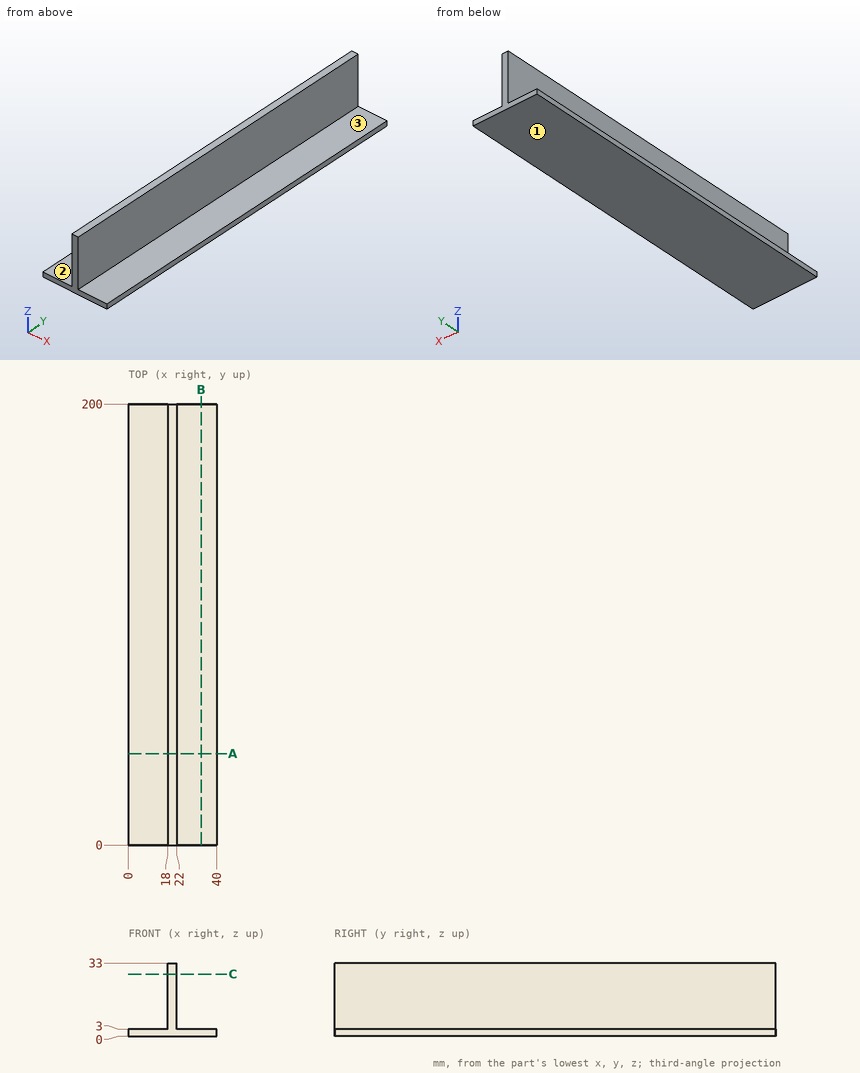
Answer from the drawing. Dimensions are ordinates in mm from the lowest x, y and z of the part. A direction names the side the tool comes from. Coordinates: 2 decimals unless noted, no trailing zeros. Write each loop counter-clockwise with the first axis right and the second up, starting at its lowest first coordinate (ties: lowest second). Pieces come first, ordered by that corner, then holes. Notation, with made-up numbers: M 47.25,41 L 104.25,41 A21 cw 104.25,66 Z; hole C 25,-25 d10. An arc over 180 degrees is marked long. Put each result on its own line as item: value. Start each with the question number.
1. A cutting plane is placed at C-C on z = 28. Write down the section's boundary in (x, y).
2. Consider line 1 (Z direction, x = 36.5, y = 144.5); line 2 (X direction, y = 53, z = 21). Determine where each line is inside the solid, lowest interval first. Write a range as from..to.
3. Which of the six approach directions +Z, -Z, +X, -X, +Y, -Y give full straight-line access (tool end or side, diameter ignored) to the marked faces 1, 2 and 3?
4. A cutting plane is placed at A-A on y = 41.5. Write down the section's boundary in (x, z), then the cut area to 3 significant figures.
5. Flat-ended cylindrical pins translate along their axes: P1, Ø5.5, axis at x = 34.5, y = 125, coming from the +Z side; P2, Ø10, axis at y = 21, z = 23, coming from the -X side. Find the tip coordinate at first contact, or state that the pin passes through.
6. A cutting plane is placed at B-B on x = 33. Write down the section's boundary in (y, z).
Resolved:
1. outline: M 18,0 L 22,0 L 22,200 L 18,200 Z
2. line 1: z = 0..3
2. line 2: x = 18..22
3. face 1: -Z, +X, -X, +Y, -Y
3. face 2: +Z, -X, +Y, -Y
3. face 3: +Z, +X, +Y, -Y
4. outline: M 0,0 L 40,0 L 40,3 L 22,3 L 22,33 L 18,33 L 18,3 L 0,3 Z
4. area: 240 mm2
5. P1: stops at z = 3
5. P2: stops at x = 18
6. outline: M 0,0 L 200,0 L 200,3 L 0,3 Z
